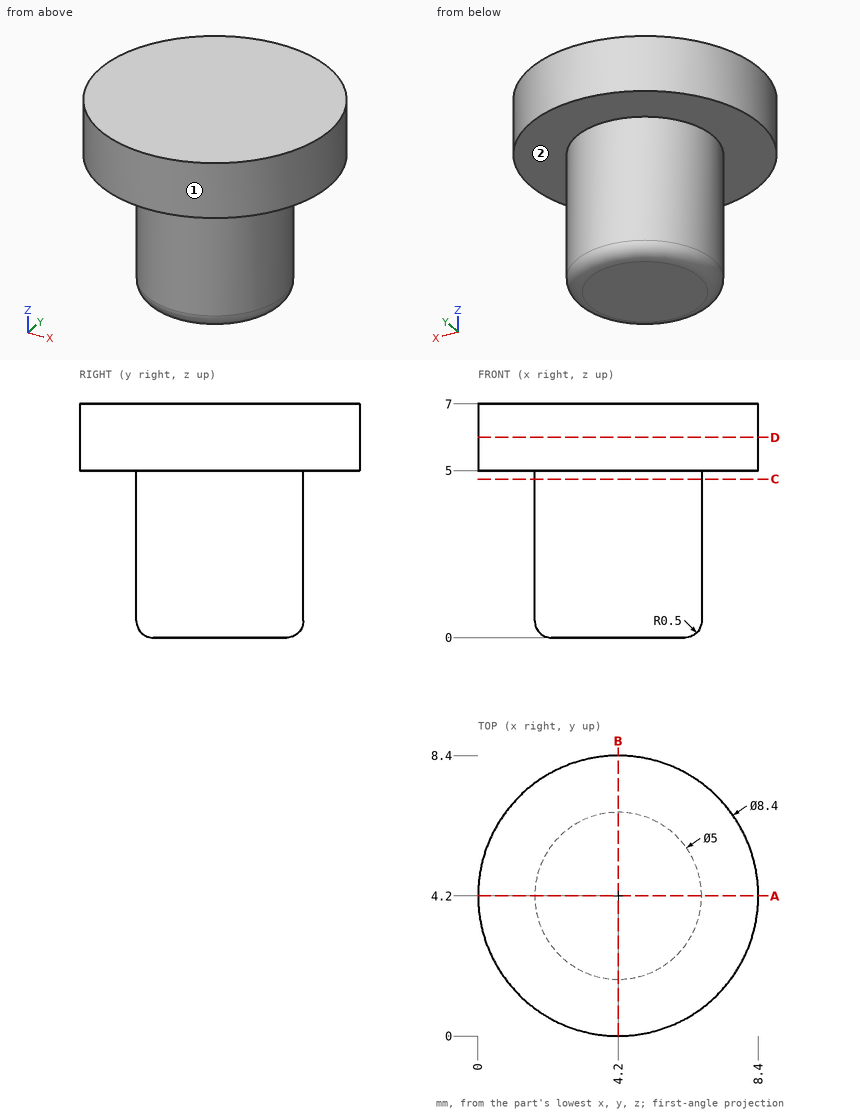
Geometry: see drawing. Coordinates: mm, zero at the bounding-box minimum. A direction names the side the tool comes from. Round coordinates to 2 decimals unless told otherwise and drop trailing zeros. Write each loop counter-clockwise with the first axis right and the second up, starting at its lowest first coordinate (ties: lowest second). Pieces come first, ordered by that corner, then holes. Notation, with made-up numbers: M 78.25,-5.75 L 87.25,-5.75 A5 cw 87.25,3.25 Z; hole C 73,17 d9. An arc over 180 degrees is marked long. Answer in a Markdown table with one row per item. Add a question column.
(1) Contact query for flat-ended pins moving along their axis: pin 1 (2 mm diameter, centred on y = 1.5, z = 1.5, fed in from +X); pin 2 (4 mm diameter, centred on x = 2, z = 6, fed in from +Y). Output: stop coordinate, or through.
(2) Cut plane A-A, the plane y = 4.2. Return the cut outline in (x, z), then the cut area to 3 significant figures.
(3) Reachability of the marked faces 1 and 2 from +Z, -Z, +X, -X, +Y, -Y: full face, straight path, thin tool, end or side. Return the list, or none.
(4) Cut plane D-D, the plane z = 6. Return the cut outline in (x, y).
(5) Ray query, L1, parallel to Z at x = 3, y = 1.25; L2, parallel to X at y = 3.75, z = 6; L3, parallel to X at y = 2.25, z = 3.25. Return the intervals inside material, ascending.
(6) Cut plane C-C, the plane z = 4.75. Return the cut outline in (x, y).
Established:
| question | item | result |
|---|---|---|
| 1 | pin 1 | x = 6.03 |
| 1 | pin 2 | y = 8.4 |
| 2 | outline | M 0,5 L 1.7,5 L 1.7,0.5 A0.5 ccw 2.2,0 L 6.2,0 A0.5 ccw 6.7,0.5 L 6.7,5 L 8.4,5 L 8.4,7 L 0,7 Z |
| 2 | area | 41.7 mm² |
| 3 | face 1 | +Z, -Z |
| 3 | face 2 | -Z |
| 4 | outline | C 4.2,4.2 d8.4 |
| 5 | L1 | 5 to 7 |
| 5 | L2 | 0.02 to 8.38 |
| 5 | L3 | 2.64 to 5.76 |
| 6 | outline | C 4.2,4.2 d5 |
